from build123d import *

# Parameters (mm, degrees)
TUBE_PROFILE_R   = 3.175
TUBE_PROFILE_R_2 = 2.175


with BuildPart() as part:
    # Tube: sweep along a curve in space
    with BuildLine() as tube_path:
        Line((154, 167, 70), (179, 167, 70))
        ThreePointArc((185, 161, 70), (183.242640687, 165.242640687, 70), (179, 167, 70))
        Line((185, 161, 70), (185, 86, 70))
        ThreePointArc((185, 80, 64), (185, 81.757359313, 68.242640687), (185, 86, 70))
        Line((185, 80, 64), (185, 80, 12))
    # Tube profile (on start of the path) → Tube (sweep)
    with BuildSketch(Plane(origin=(154, 167, 70), x_dir=(0, 0, 1), z_dir=(1, 0, 0))):
        Circle(TUBE_PROFILE_R)
        Circle(TUBE_PROFILE_R_2, mode=Mode.SUBTRACT)
    sweep(path=tube_path.line)


solid = part.part
Here's how the part is built. I have some questions about the finished solid (model axes, mm). A direction names the side the tool comes from. Coordinates: 2 decimals unless noted, no trailing zeros. Order: outer loops, then holes, each group sorted by start corner. A loop starts at its lowest first (then second) coordinate and runs counter-clockwise, first axis right, second up. Notation, with made-up numbers: M -30,0 L -14,0 A23 ccw -14,22 Z; hole C -10.75,-14 d5. An arc over 180 degrees is marked long. Answer as CSV lines item,"result". Start each with the question number.
1. We'd pull the mould along Y, two halves only. Please class faces 1 (the flat face through (154, 169.1, 71.4)), 2 (the cylindrical face through (166.68, 166.05, 73.03)), 3 (the cylindrical face through (184.05, 122.98, 73.03)): released by +Y, released by -Y, zero draft, split by the parting line, or undercut.
2. I need wall thicknesses on line 1 (Z direction, x = 185, y = 103) (3 decimals); line 2 (X direction, y = 80, z = 42) (3 decimals); line 3 (X direction, y = 112.5, z = 69). Which ranges of each line are inside material? Lowest first, please. Write a range as [from, to].
3. On a 3-axis mill with a long thin cutter (end or side, diameter ignored), from which of +Z, -Z, +X, -X, +Y, -Y can I reach the whole of each face in a straight line? I mean faces 4 (the cylindrical face through (184.347, 122.975, 72.075)), 5 (the cylindrical face through (183.166, 78.831, 37.636)), 6 (the cylindrical face through (166.675, 165.166, 71.169)). Say none if no direction works.
4. For pin 1 (5 mm diameter, centred on x = 185, z = 70, fed in from -Y); pin 2 (7 mm diameter, centred on y = 167, z = 70, fed in from +X); pin 3 (2.5 mm diameter, centred on x = 185, y = 80, fed in from +Z); pin 4 (10 mm diameter, centred on x = 173, z = 55, fed in from +Y), each with a flat end and sliding along its axis, tell me the tip position at first contact or that it passes through.
5. I want a section at B-B, the plane y = 97.5. Write out the boundary of the cut face in (x, z) (3 decimals), and give its area (3 significant figures).
6. I want a section at A-A, the plane z = 30.5. Write out the boundary of the cut face in (x, y) (3 decimals), and give its area (3 significant figures).
Recorded:
1,face 1,"zero draft"
1,face 2,"split by the parting line"
1,face 3,"undercut"
2,line 1,"z = [66.825, 67.825], [72.175, 73.175]"
2,line 2,"x = [181.825, 182.825], [187.175, 188.175]"
2,line 3,"x = [181.99, 183.07], [186.93, 188.01]"
3,face 4,"none"
3,face 5,"-Z"
3,face 6,"-X"
4,pin 1,"stops at y = 77.52"
4,pin 2,"stops at x = 187.83"
4,pin 3,"stops at z = 71.85"
4,pin 4,"passes through"
5,outline,"C 185,70 d6.35; hole C 185,70 d4.35"
5,area,"16.8 mm2"
6,outline,"C 185,80 d6.35; hole C 185,80 d4.35"
6,area,"16.8 mm2"
